Build history of the part. All positions in model axes, mm. A direction names the side the tool comes from. Round coordinates to 2 decimals unless told otherwise and drop trailing zeros. Write each loop counter-clockwise with the first axis right and the second up, starting at its lowest first coordinate (ties: lowest second). Pieces come first, ordered by that corner, then holes.
1) Saw through at C-C (z = 14). Write the cut outline in (x, y) (3 decimals), plus the area to 3 significant figures.
2) Saw through at A-A (z = 34.5). Write the cut outline in (x, y) (3 decimals), plus the area to 3 significant figures.
3) Flat gauge pins, fed straight in: pin 1 (1.5 mm diameter, centred on y = 48, z = 11, fed in from +X); pin 2 (12 mm diameter, centred on x = -7.5, y = 31, fed in from -Z); pin 3 (12 mm diameter, centred on x = 27.38, y = 42.88, fed in from -Z). Where does each tip first touch, or does it go through?
4) Pull direction X, two halves, no side cores. Call faces 3 (the flat face through (30.33, 29, 27.82)), 4 (the flat face through (-30.33, 29, 27.82)), 5 (the cylindrical face through (-31.19, 46.38, 21.08)): +X half, -X half, draft (parallel to the pull), parting line (faces both ways), or undercut.
5) Saw through at B-B (y = 41.5). State how many separate pieces and enclosed holes the cut face has, plus the area to 3 significant figures.
6) Which spindle directions (+Z, -Z, +X, -X, +Y, -Y) get a long thin tool onto all of the face, cutting with end or side? Do faces 1 (the cylindrical face through (30.157, 47.246, 21.076)), 2 (the flat face through (-0.1, 36.3, 15.427)). Say none if no direction does.
7) Wall check: probe 1 along X at (y, z) = (39.25, 22); probe 2 along X at (y, z) = (45.25, 14); probe 3 along X at (y, z) = (33.25, 31.5). Give the ranges that are in metal, low to high.
from build123d import *

# Parameters (mm, degrees)
SKETCH004_R  = 5.175
PAD002_DEPTH = 41.4


with BuildPart() as chamfer_cutout_left:
    # Sketch005 → Revolution001 (revolve)
    with BuildSketch(Plane.YZ):
        with BuildLine():
            Line((36.1, 15.427249), (39.9, 15.427249))
            ThreePointArc((39.9, 15.427249), (48.355241, 6.793042), (58.35, 0))
            Line((58.35, 0), (58.35, -5))
            Line((58.35, -5), (36.1, -5))
            Line((36.1, -5), (36.1, 15.427249))
        make_face()
    revolve(axis=Axis((0, 0, 0), (0, 0, 1)))


with BuildPart() as spacer_left:
    # Sketch004 → Pad002 (new body)
    with BuildSketch(Plane.XY):
        with BuildLine():
            ThreePointArc((-15.484484, 45.433806), (-31.397174, 49.18272), (-34.694729, 33.170405))
            Line((-26.093327, 24.946909), (-34.694729, 33.170405))
            ThreePointArc((26.093327, 24.946909), (0, 36.1), (-26.093327, 24.946909))
            Line((26.093327, 24.946909), (34.694729, 33.170405))
            ThreePointArc((34.694729, 33.170405), (31.397174, 49.18272), (15.484484, 45.433806))
            ThreePointArc((15.484484, 45.433806), (0, 48), (-15.484484, 45.433806))
        make_face()
        with Locations((-27.375, 42.882106)):
            Circle(SKETCH004_R, mode=Mode.SUBTRACT)
        with Locations((27.375, 42.882106)):
            Circle(SKETCH004_R, mode=Mode.SUBTRACT)
    extrude(amount=PAD002_DEPTH)

    # Cut001: cut chamfer_cutout_left
    add(chamfer_cutout_left.part, mode=Mode.SUBTRACT)


solid = spacer_left.part
Evaluation:
1. outline: (-34.695, 33.17) - (-29.693, 28.388) arc R41.08 cw to (29.693, 28.388) - (34.695, 33.17) arc R11.4 ccw (long way) to (15.484, 45.434) arc R48 ccw to (-15.484, 45.434) arc R11.4 ccw (long way) to start; hole circle Ø10.35 at (-27.375, 42.882); hole circle Ø10.35 at (27.375, 42.882)
1. area: 711 mm2
2. outline: (-34.695, 33.17) - (-26.093, 24.947) arc R36.1 cw to (26.093, 24.947) - (34.695, 33.17) arc R11.4 ccw (long way) to (15.484, 45.434) arc R48 ccw to (-15.484, 45.434) arc R11.4 ccw (long way) to start; hole circle Ø10.35 at (-27.375, 42.882); hole circle Ø10.35 at (27.375, 42.882)
2. area: 1,020 mm2
3. pin 1: stops at x = 33.69
3. pin 2: stops at z = 15.43
3. pin 3: stops at z = 0.83
4. face 3: +X half
4. face 4: -X half
4. face 5: undercut
5. separate pieces: 3
5. enclosed holes: 0
5. area: 1,660 mm2
6. face 1: +Z, -Z
6. face 2: -Z, -Y
7. probe 1: x = -36.66 to -31.06, -23.69 to 23.69, 31.06 to 36.66
7. probe 2: x = -35.15 to -31.98, -22.77 to 22.77, 31.98 to 35.15
7. probe 3: x = -34.75 to -14.06, 14.06 to 34.75
